Check sheet for the modelled part. Datum: model origin and axes. Units: mm. Face numbers are marked on the shaded views. A direction names the side the tool comes from. Round coordinates to 2 decimals unless told otherwise and drop trailing zeros. Loops run counter-clockwise (first coordinate to the right, second up) from the corner with the lowest first, then second, coordinate; pieces in that order, holes last. Notation, with made-up numbers: (16, 62) -> (53, 62) arc R20 ccw to (53, 74) -> close; hole circle Ø1 at (-15.75, 20.5). An arc over 180 degrees is marked (long way). One line per question, with ' | ' between items.
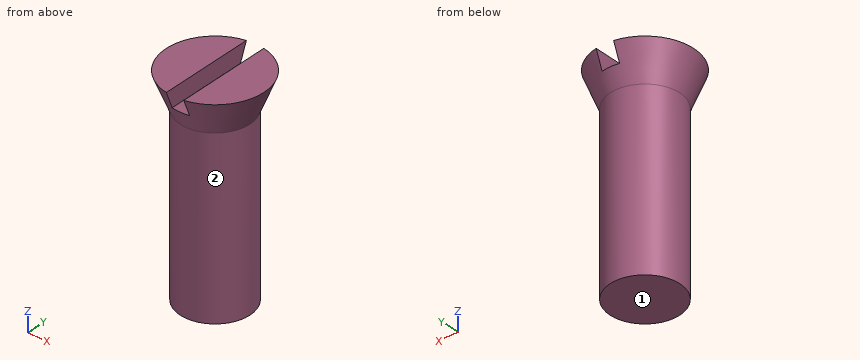
```python
from build123d import *

# Parameters (mm, degrees)
BOX_W          = 1
BOX_H          = 10
BOX_DEPTH      = 4
CYLINDER_R     = 2
CYLINDER_DEPTH = 10


with BuildPart() as cub:
    # Box → Box (new body)
    with BuildSketch(Plane(origin=(-0.5, -6, 11), x_dir=(1, 0, 0), z_dir=(0, 0, 1))):
        with Locations((0.5, 5)):
            Rectangle(BOX_W, BOX_H)
    extrude(amount=BOX_DEPTH)


with BuildPart() as cilindre:
    # Cylinder → Cylinder (new body)
    with BuildSketch(Plane.XY):
        Circle(CYLINDER_R)
    extrude(amount=CYLINDER_DEPTH)


with BuildPart() as cut:
    # Cone → Cone (revolve)
    with BuildSketch(Plane(origin=(0, 0, 10), x_dir=(1, 0, 0), z_dir=(0, -1, 0))):
        Polygon((0, 0), (2, 0), (2.8, 2), (0, 2), align=None)
    revolve(axis=Axis((0, 0, 10), (0, 0, 1)))

    # Fusion: union Cilindre
    add(cilindre.part)

    # Cut: cut Cub
    add(cub.part, mode=Mode.SUBTRACT)


solid = cut.part
```
(1) Go/stop test with flat-tipped pins: pin 1 (0.5 mm diameter, centred on x = 0, y = -0.5, fed in from +Z); pin 2 (3 mm diameter, centred on x = -2, z = 8.5, fed in from -Y); pin 3 (2 mm diameter, centred on x = -2, z = 1.5, fed in from -Y). Record where each tip stops, or that it passes through.
Answer:
pin 1: stops at z = 11 | pin 2: stops at y = -1.94 | pin 3: stops at y = -1.73
(2) Sectioned sample at B-B, the plane x = 0. Record the cut outline in (y, z), and give its area (3 significant figures).
Answer:
outline: (-2.4, 11) -> (-2, 10) -> (-2, 0) -> (2, 0) -> (2, 10) -> (2.4, 11) -> close | area: 44.4 mm2
(3) Sectioned sample at A-A, the plane y = 0. Record the cut outline in (x, z).
Answer:
outline: (-2.8, 12) -> (-2, 10) -> (-2, 0) -> (2, 0) -> (2, 10) -> (2.8, 12) -> (0.5, 12) -> (0.5, 11) -> (-0.5, 11) -> (-0.5, 12) -> close
(4) Set-up check for the marked faces 1 and 2: record each of +Z, -Z, +X, -X, +Y, -Y from which the full face is reachable in a straight line by a thin tool's end or side.
Answer:
face 1: -Z, +X, -X, +Y, -Y | face 2: -Z
(5) Sectioned sample at C-C, the plane z = 7. Record the cut outline in (x, y), and give its area (3 significant figures).
Answer:
outline: circle Ø4 at (0, 0) | area: 12.6 mm2
(6) Scan lines: probe 1 along Z at (x, y) = (0.3, -0.75); probe 2 along Y at (x, z) = (-0.1, 1); probe 3 along X at (y, z) = (2.25, 11.25). Record each from-to range of solid material in increasing order.
Answer:
probe 1: z = 0 to 11 | probe 2: y = -2 to 2 | probe 3: x = -1.09 to -0.5, 0.5 to 1.09
